The model under review builds one solid part; all positions refer to its coordinate system, in mm. Face numbers are marked on the shaded views. A direction names the side the tool comes from. Round coordinates to 2 decimals unless told otherwise and drop trailing zeros. Loops run counter-clockwise (first coordinate to the right, second up) from the corner with the lowest first, then second, coordinate; pieces in that order, holes last. Notation, with made-up numbers: M -29.75,-22 L 8.25,-22 A26 cw 8.25,-4 Z; hole C 73.25,34 d2. An arc over 180 degrees is marked long. Answer as a JSON object with one key per item and string values. Group by question number.
Item 1: Insertion check: P1, Ø3, axis at x = 11.5, y = 4, coming from the -Z side; P2, Ø3, axis at x = 9.5, y = 6, coming from the +Z side; P3, Ø10, axis at x = 15, y = 5, coming from the -Z side; P4, Ø2, axis at x = -5, z = 4, coming from the +Y side. Each pin has a flat end and moves straight along its axis. Give the tip position at first contact, or say it passes through.
Item 2: Tool access review of the marked faces 1 and 2: name each direction out of +Z, -Z, +X, -X, +Y, -Y from which nothing blocks a thin tool from reaching the whole face with its end or side.
Item 3: To check wall thickness, follow line 1 (X direction, y = -7.25, z = 3.75); line 2 (Z direction, x = 31, y = 0); line 3 (Z direction, x = -10.5, y = -0.25). State the ranges of each line that lie inside material, in increasing order.
Item 4: Consider section A-A (y = 0). Give the boundary of the cut face in (x, z) (3 decimals), and give its area (3 significant figures).
Item 5: Consider section D-D (z = -7). Give the boundary of the cut face in (x, y).
Item 6: Consider section C-C (z = 7.25). Give the boundary of the cut face in (x, y).
Item 7: Consider section B-B (x = -14.5). Give the boundary of the cut face in (y, z).
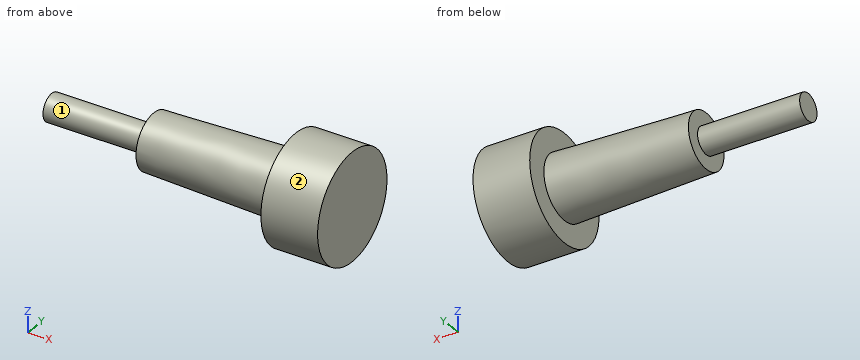
```python
from build123d import *

# Parameters (mm, degrees)
F0_R     = 4.953
F2_R     = 5.715
F4_R     = 2.413
F5_DEPTH = 18.288
F6_R     = 9.652
F6_R_2   = 5.715
F7_DEPTH = 10.16


with BuildPart() as f3:
    # F0 (on Right) → F3 section 0
    with BuildSketch(Plane.YZ):
        Circle(F0_R)
    # F2 (on offset) → F3 section 1
    with BuildSketch(Plane.YZ.offset(25.4)):
        Circle(F2_R)
    loft()

    # F4 (on face) → F5 (join)
    with BuildSketch(Plane(origin=(0, 0, 0), x_dir=(0, -1, 0), z_dir=(-1, 0, 0))):
        Circle(F4_R)
    extrude(amount=F5_DEPTH)

    # F6 (on face) → F7 (join)
    with BuildSketch(Plane.YZ.offset(25.4)):
        Circle(F6_R)
        Circle(F6_R_2, mode=Mode.SUBTRACT)
        Circle(F6_R_2)
    extrude(amount=F7_DEPTH)


solid = f3.part
```
Geometry results:
{
 "1": {"P1": "stops at z = -4.67", "P2": "stops at z = 2.68", "P3": "stops at z = -5.45", "P4": "passes through"},
 "2": {"face 1": "-X", "face 2": "+X, -X"},
 "3": {"line 1": "x = 25.4 to 35.56", "line 2": "z = -9.65 to 9.65", "line 3": "z = -2.4 to 2.4"},
 "4": {"outline": "M -18.288,-2.413 L 0,-2.413 L 0,-4.953 L 25.4,-5.715 L 25.4,-9.652 L 35.56,-9.652 L 35.56,9.652 L 25.4,9.652 L 25.4,5.715 L 0,4.953 L 0,2.413 L -18.288,2.413 Z", "area": "555 mm^2"},
 "5": {"outline": "M 25.4,-6.65 L 35.56,-6.65 L 35.56,6.65 L 25.4,6.65 Z"},
 "6": {"outline": "M 25.4,-6.37 L 35.56,-6.37 L 35.56,6.37 L 25.4,6.37 Z"},
 "7": {"outline": "C 0,0 d4.83"}
}
